Part print with two shaded views. Sizes in mm from the minimum x, y, z corner. A direction names the side the tool comes from. Round coordinates to 2 decimals unless told otherwise and drop trailing zeros. Write each loop counter-clockwise with the first axis right and the second up, starting at its lowest first coordinate (ties: lowest second). Pieces come first, ordered by that corner, then holes. Notation, with made-up numbers: (31.5, 2.5) - (83.5, 2.5) arc R23 cw to (83.5, 34.5) - close; hole circle Ø11 at (56, 68.25). An arc over 180 degrees is marked (long way). Answer as a JSON object with one key per item and string values. Group by question number.
Item 1: Two-plate mould, pull along X, no slides. Class the marked faces 4, 5, 6 and 7: +X half, -X half, draft (parallel to the pull), parting line (faces both ways), or undercut.
Item 2: Slice it at B-B, the plane x = 7. List the corners of the cut face in (y, z).
Item 3: Slice it at D-D, the plane z = 7. List the corners of the cut face in (x, y), then the cut area to 3 significant figures.
Item 4: Probe line 1 (Y direction, x = 7, z = 5); line 2 (X direction, y = 5, z = 3.75); line 3 (Y direction, x = 5.5, z = 2.5). List the from-to ranges inside material, lowest first. Write a range as from..to.
Item 5: Slice it at A-A, the plane y = 34. List the corners of the cut face in (x, z).
Item 6: Slice it at C-C, the plane z = 1. List the corners of the cut face in (x, y), then the cut area to 3 significant figures.
Item 7: Which spindle directions (+Z, -Z, +X, -X, +Y, -Y) get a long thin tool onto all of the face, cutting with end or side? Do the marked faces 1, 2 and 3. Say none if no direction does.
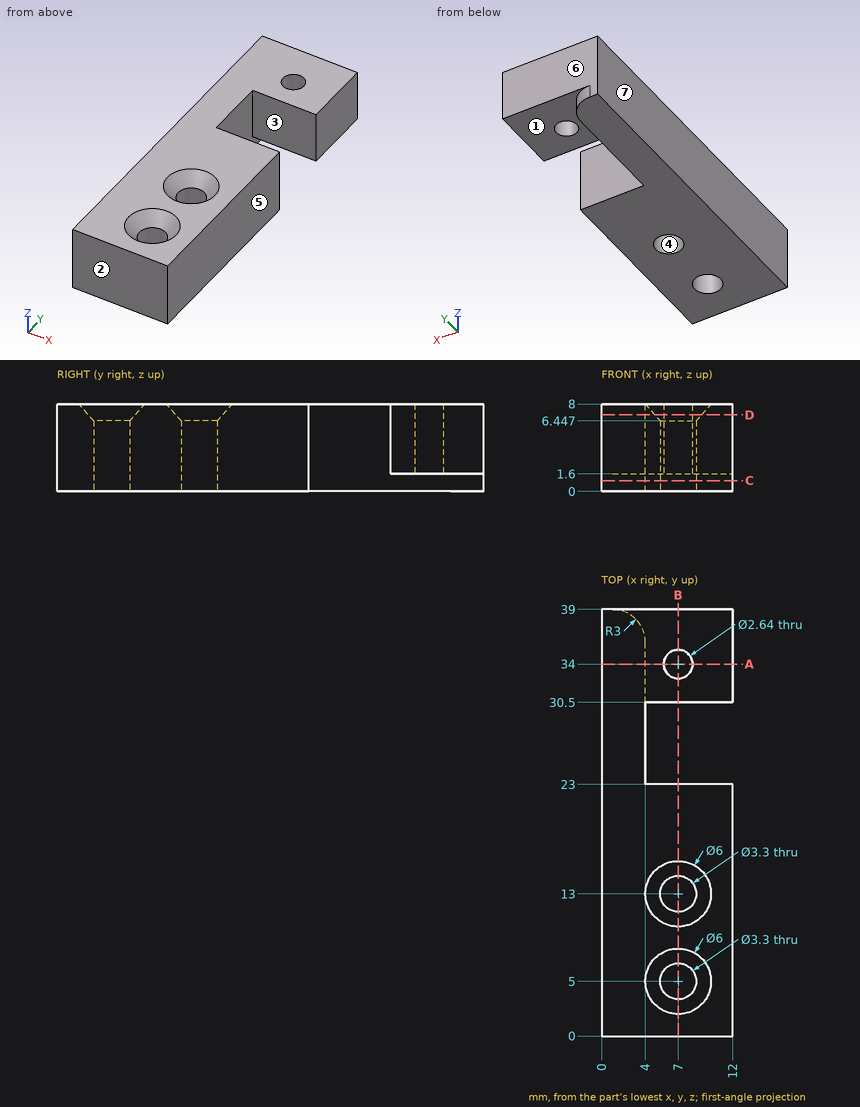
Geometry says:
{
 "1": {"face 4": "undercut", "face 5": "+X half", "face 6": "draft", "face 7": "-X half"},
 "2": {"outline": "(0, 0) - (3.35, 0) - (3.35, 6.45) - (2, 8) - (0, 8) - close; (6.65, 0) - (11.35, 0) - (11.35, 6.45) - (10, 8) - (8, 8) - (6.65, 6.45) - close; (14.65, 0) - (23, 0) - (23, 8) - (16, 8) - (14.65, 6.45) - close; (30.5, 1.6) - (32.68, 1.6) - (32.68, 8) - (30.5, 8) - close; (35.32, 1.6) - (39, 1.6) - (39, 8) - (35.32, 8) - close"},
 "3": {"outline": "(0, 0) - (12, 0) - (12, 23) - (4, 23) - (4, 30.5) - (12, 30.5) - (12, 39) - (0, 39) - close; hole circle Ø4.26 at (7, 5); hole circle Ø4.26 at (7, 13); hole circle Ø2.64 at (7, 34)", "area": "374 mm^2"},
 "4": {"line 1": "y = 0..3.35, 6.65..11.35, 14.65..23, 30.5..32.68, 35.32..39", "line 2": "x = 0..5.35, 8.65..12", "line 3": "y = 0..4.31, 5.69..12.31, 13.69..23, 30.5..39"},
 "5": {"outline": "(0, 0) - (4, 0) - (4, 1.6) - (5.68, 1.6) - (5.68, 8) - (0, 8) - close; (8.32, 1.6) - (12, 1.6) - (12, 8) - (8.32, 8) - close"},
 "6": {"outline": "(0, 0) - (12, 0) - (12, 23) - (4, 23) - (4, 36) arc R3 ccw to (1, 39) - (0, 39) - close; hole circle Ø3.3 at (7, 5); hole circle Ø3.3 at (7, 13)", "area": "321 mm^2"},
 "7": {"face 1": "-Z, +X, +Y", "face 2": "+Z, -Z, +X, -X, -Y", "face 3": "+Z, -Z, +X"}
}
